Source: CAD feature listing. Evaluate the final solid. Frame: model axes, mm. Round coordinates to 2 decimals unless told otherwise and drop trailing zeros. Order: outer loops, then holes, each group sorted by start corner. A loop starts at its lowest first (then second) coordinate and runs counter-clockwise, first axis right, second up. Notation, with made-up numbers: M 50.25,77 L 72.25,77 A30 ccw 72.25,112 Z; hole C -14,87.5 d11. An arc over 180 degrees is marked long. Answer in a Markdown table with one row per item. Add a question column.
```python
from build123d import *

# Parameters (mm, degrees)
SKETCH017_R  = 1.55
PAD014_DEPTH = 0.75
FILLET020_R  = 0.4
FILLET021_R  = 1


with BuildPart() as part:
    # Sketch017 → Pad014 (new body, symmetric)
    with BuildSketch(Plane.XZ):
        with BuildLine():
            Line((-20, 20), (-20, -17))
            Line((-20, -18.5), (-20, -17))
            Line((-20, -18.5), (-20, -20))
            Line((-20, -20), (20, -20))
            Line((20, -20), (20, 14))
            Line((18.133975, 14.5), (20, 14))
            Line((18.133975, 14.5), (-14.2, 14.5))
            ThreePointArc((-15, 14.5), (-14.6, 14.1), (-14.2, 14.5))
            Line((-15, 14.5), (-15, 15.2))
            ThreePointArc((-15, 16), (-15.4, 15.6), (-15, 15.2))
            Line((-15, 16), (18.133975, 16))
            Line((18.133975, 16), (20, 16.5))
            Line((20, 16.5), (20, 20))
            Line((20, 20), (-20, 20))
        make_face()
        with Locations((0, 10)):
            Circle(SKETCH017_R, mode=Mode.SUBTRACT)
        with Locations((0, -10)):
            Circle(SKETCH017_R, mode=Mode.SUBTRACT)
    extrude(amount=PAD014_DEPTH, both=True)

    # Fillet020
    fillet020_edges = [part.edges().sort_by_distance(p)[0] for p in [
        (-15, 0, 15.2),
        (-14.2, 0, 14.5),
    ]]
    fillet(fillet020_edges, radius=FILLET020_R)

    # Fillet021
    fillet021_edges = [part.edges().sort_by_distance(p)[0] for p in [
        (-20, 0, 20),
        (-20, 0, -20),
        (20, 0, -20),
        (20, 0, 14),
        (18.133975, 0, 14.5),
        (18.133975, 0, 16),
        (20, 0, 16.5),
        (20, 0, 20),
    ]]
    fillet(fillet021_edges, radius=FILLET021_R)


solid = part.part
```
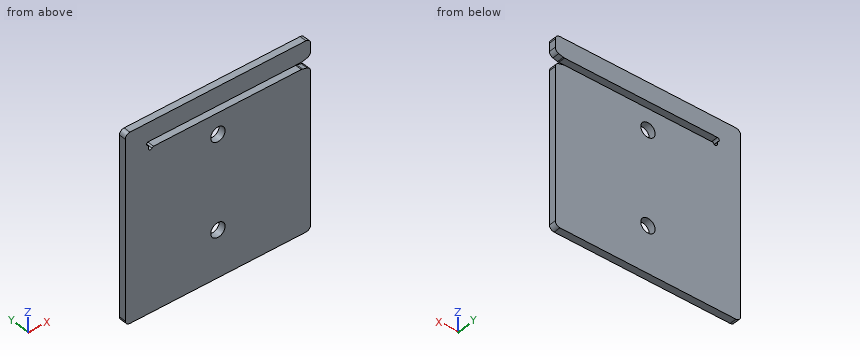
(1) Cut plane B-B (y = 0.05). Return loops of the section in (x, z).
(2) Cut plane D-D (x = 0). Return loops of the section in (y, z), and give its area (4 significant figures).
(3) Pin query (flat end, axial travel): pin 1 (4 mm diameter, centred on x = 0, z = 10, fed in from -Y). Return the tip coordinate at first contact, or that it passes through.
(4) Cut plane C-C (z = 10). Return loops of the section in (x, y), and give its area (4 significant figures).
(5) Cut plane A-A (x = 14). Return loops of the section in (y, z), and give its area (4 significant figures).
(6) Line query: line 1 (Z direction, x = 0, y = -0.2); line 2 (Z direction, x = 16, y = 0.3); line 3 (X direction, y = 0, z = 13.5). Output: solid intervals per line, ascending. Write a range as from..to.
Answer list:
| question | item | result |
|---|---|---|
| 1 | outline | M -20,-19 A1 ccw -19,-20 L 19,-20 A1 ccw 20,-19 L 20,13.23 A1 ccw 19.26,14.2 L 18.26,14.47 A1 ccw 18,14.5 L -13.91,14.5 A0.4 ccw -14.25,14.3 A0.4 cw -15,14.5 L -15,14.91 A0.4 ccw -15.2,15.25 A0.4 cw -15,16 L 18,16 A1 ccw 18.26,16.03 L 19.26,16.3 A1 ccw 20,17.27 L 20,19 A1 ccw 19,20 L -19,20 A1 ccw -20,19 Z; hole C 0,-10 d3.1; hole C 0,10 d3.1 |
| 2 | outline | M -0.75,-20 L 0.75,-20 L 0.75,-11.55 L -0.75,-11.55 Z; M -0.75,-8.45 L 0.75,-8.45 L 0.75,8.45 L -0.75,8.45 Z; M -0.75,11.55 L 0.75,11.55 L 0.75,14.5 L -0.75,14.5 Z; M -0.75,16 L 0.75,16 L 0.75,20 L -0.75,20 Z |
| 2 | area | 48.45 mm² |
| 3 | pin 1 | y = -0.75 |
| 4 | outline | M -20,-0.75 L -1.55,-0.75 L -1.55,0.75 L -20,0.75 Z; M 1.55,-0.75 L 20,-0.75 L 20,0.75 L 1.55,0.75 Z |
| 4 | area | 55.35 mm² |
| 5 | outline | M -0.75,-20 L 0.75,-20 L 0.75,14.5 L -0.75,14.5 Z; M -0.75,16 L 0.75,16 L 0.75,20 L -0.75,20 Z |
| 5 | area | 57.75 mm² |
| 6 | line 1 | -20..-11.55, -8.45..8.45, 11.55..14.5, 16..20 |
| 6 | line 2 | -20..14.5, 16..20 |
| 6 | line 3 | -20..19.96 |
